Design review of the part shown in the three views and the two pictorial views. Dimensions are in mm from the part's minimum x, y and z. A direction names the side the tool comes from. Give positions to 0.01 mm unless a question says otherwise; leave off trailing zeros. Loops run counter-clockwise (first coordinate to the right, second up) from the corner with the lowest first, then second, coordinate; pieces in that order, holes last. Notation, with made-up numbers: (49.25, 70.25) - (91.25, 70.25) arc R27 ccw to (91.25, 96.25) - close; hole circle Ø4 at (62, -27.75). An arc over 180 degrees is marked (long way). Answer as a JSON object with one key per item and string values.
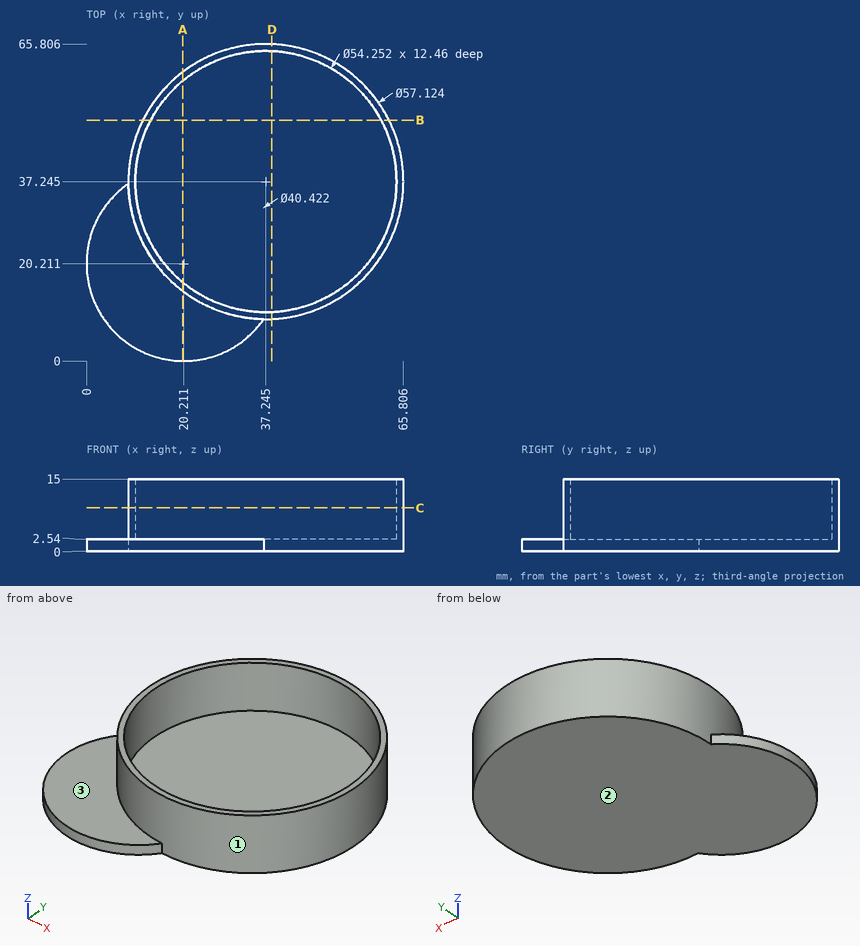
Q1. Consider section C-C, the plane z = 9. State the section outline as (x, y) points (1 decimal).
Results:
{"outline": "circle Ø57.1 at (37.2, 37.2); hole circle Ø54.3 at (37.2, 37.2)"}
Q2. To check wall thickness, follow probe 1 along Z at (x, y) = (42, 25.5); probe 2 along Y at (x, z) = (15.5, 4.5) (1 decimal); probe 3 along Y at (x, z) = (30.5, 4). State the ranges of each line that lie inside material, in increasing order. Write a range as [from, to].
Results:
{"probe 1": "z = [0, 2.54]", "probe 2": "y = [18.7, 21], [53.5, 55.8]", "probe 3": "y = [9.49, 10.97], [63.52, 65]"}
Q3. For the marked faces 1, 2 and 3, list the 3-axis set-ups (+Z, -Z, +X, -X, +Y, -Y) from which the entire face can be reached by the end or side of a thin tool; tool diameter is ignored.
Results:
{"face 1": "+Z", "face 2": "-Z, +X, -X, +Y, -Y", "face 3": "+Z, -X, -Y"}
Q4. Consider section D-D, the plane x = 38.5. State the section outline as (y, z) points, plus the area to 3 significant figures.
Results:
{"outline": "(8.71, 0) - (65.78, 0) - (65.78, 15) - (64.34, 15) - (64.34, 2.54) - (10.15, 2.54) - (10.15, 15) - (8.71, 15) - close", "area": "181 mm^2"}
Q5. Consider section A-A, the plane x = 20. State the section outline as (y, z) points, plus the area to 3 significant figures.
Results:
{"outline": "(0, 0) - (60.01, 0) - (60.01, 15) - (58.18, 15) - (58.18, 2.54) - (16.31, 2.54) - (16.31, 15) - (14.48, 15) - (14.48, 2.54) - (0, 2.54) - close", "area": "198 mm^2"}
Q6. Consider section B-B, the plane y = 50. State the section outline as (x, z) points (1 decimal), plus the area to 3 significant figures.
Results:
{"outline": "(11.7, 0) - (62.8, 0) - (62.8, 15) - (61.2, 15) - (61.2, 2.5) - (13.3, 2.5) - (13.3, 15) - (11.7, 15) - close", "area": "170 mm^2"}
Q7. Clearance check with flat-ended pins moving along their axes: pin 1 Ø3 at (y, z) = (46.5, 2.5) entering from -X; pin 2 Ø3 at (x, z) = (47.5, 12) entering from -Y; pin 3 Ø3 at (x, z) = (44, 11) entering from -Y. State where each tip first meets the part, or that it passes through.
Results:
{"pin 1": "stops at x = 9.76", "pin 2": "stops at y = 10.06", "pin 3": "stops at y = 9.17"}
